Study the drawing (mm; zero at the part's minimum x, y, z) and answer. Coordinates: 2 decimals unless noted, no trailing zeros. Write each loop counter-clockwise with the first axis right and the second up, starting at its lowest first coordinate (ties: lowest second). Pieces come first, ordered by that corner, then holes. Notation, with made-up numbers: (70, 54) - (86, 54) arc R27 ccw to (86, 79) - close; hole circle Ø3 at (-1, 82). An arc over 180 degrees is marked (long way). One line per item, written item: value.
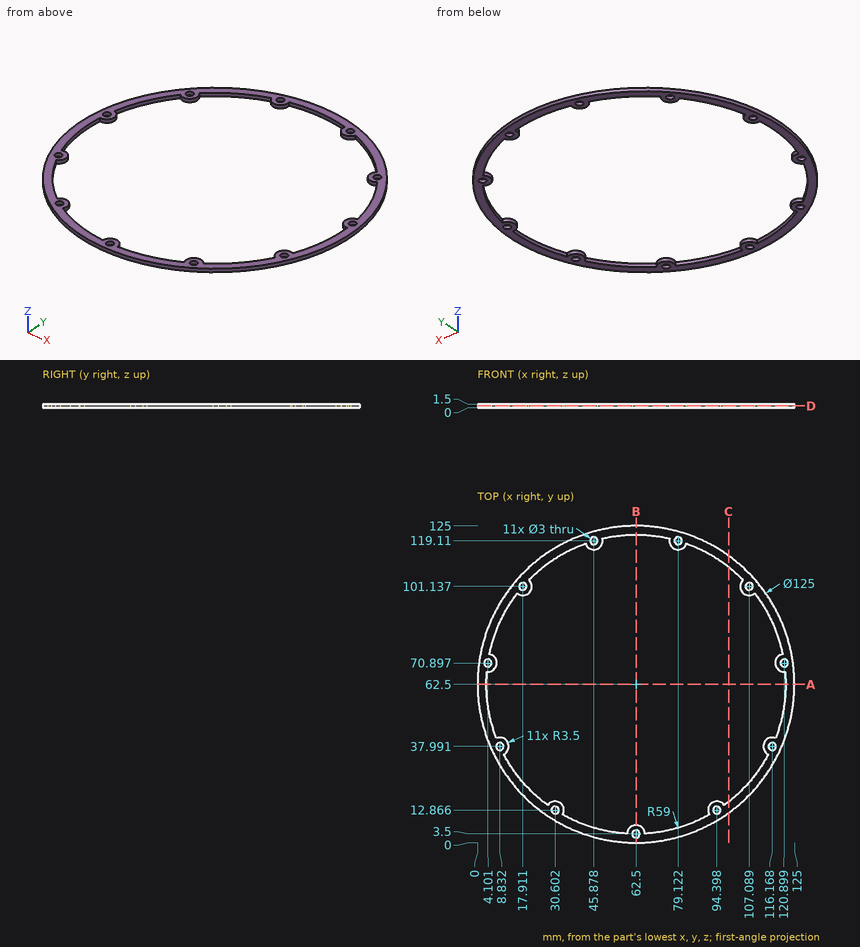
Item 1: Section A-A, the plane y = 62.5 is taken. Determine the outline of the cut face in (x, z), then the cut area to 3 significant figures.
Evaluation:
outline: (0, 0) - (3.5, 0) - (3.5, 1.5) - (0, 1.5) - close; (121.5, 0) - (125, 0) - (125, 1.5) - (121.5, 1.5) - close
area: 10.5 mm2
Item 2: Section C-C, the plane x = 99 is taken. Determine the outline of the cut face in (y, z) (1 decimal).
Evaluation:
outline: (11.8, 0) - (16.1, 0) - (16.1, 1.5) - (11.8, 1.5) - close; (108.9, 0) - (113.2, 0) - (113.2, 1.5) - (108.9, 1.5) - close
Item 3: Consider probe 1 along X at (y, z) = (11.5, 0.1) (1 decimal); probe 2 along Y at (x, z) = (106, 1.45) (1 decimal); probe 3 along X at (y, z) = (44.5, 1). Determine where each line is inside the solid, lowest interval first.
Evaluation:
probe 1: x = 26.4 to 30, 31.2 to 33.8, 91.2 to 93.8, 95 to 98.6
probe 2: y = 17.6 to 22.6, 97.8 to 100.1, 102.2 to 107.4
probe 3: x = 2.65 to 6.31, 118.69 to 122.35
Item 4: Section B-B, the plane x = 62.5 is taken. Determine the outline of the cut face in (y, z).
Evaluation:
outline: (0, 0) - (2, 0) - (2, 1.5) - (0, 1.5) - close; (5, 0) - (7, 0) - (7, 1.5) - (5, 1.5) - close; (121.5, 0) - (125, 0) - (125, 1.5) - (121.5, 1.5) - close
Item 5: Given pin 1 (5 mm diameter, centred on x = 79.12, y = 119.11, fed in from -Z), flat-ended and moving along its own axis, determine where the tip first touches the part or whether it passes through.
Evaluation:
pin 1: stops at z = 0
Item 6: Section D-D, the plane z = 0.8 is taken. Give the number of separate pieces and of enclosed holes in the cut face, then the cut area to 3 significant figures.
Evaluation:
separate pieces: 1
enclosed holes: 12
area: 1,470 mm2
